Design review of the part built by this model. Coordinates are the model's own, in mm. A direction names the side the tool comes from. Give positions to 0.01 mm unless a question says otherwise; leave off trailing zeros. Order: outer loops, then holes, each group sorted by start corner. A loop starts at its lowest first (then second) coordinate and runs counter-clockwise, first axis right, second up. Notation, with made-up numbers: (86.25, 86.25) - (114.25, 86.25) arc R13 cw to (114.25, 93.25) - close; hole circle Ø7 at (45, 55). An arc over 180 degrees is marked (long way). Write each question's results on one line, items separated by ' | '. Start each with the question number.
Autodesk Inventor part; units mm, degrees
ref_plane "YZ Plane" through (0, 0, 0) normal (1, 0, 0) x (0, 1, 0)
ref_plane "XZ Plane" through (0, 0, 0) normal (0, 1, 0) x (-1, 0, 0)
ref_plane "XY Plane" through (0, 0, 0) normal (0, 0, 1) x (1, 0, 0)
sketch "Skizze1" plane through (0, 0, 0) normal (0, 0, 1) x (1, 0, 0)
  line L0 (-40, -9) -> (40, -9)
  line L1 (40, -9) -> (40, 9)
  line L2 (40, 9) -> (-40, 9)
  line L3 (-40, 9) -> (-40, -9)
  line L4 (-40, -9) -> (40, 9) construction
  line L5 (40, -9) -> (-40, 9) construction
  point P0 (0, 0)
  dimension "Breite" = 80
  dimension "Höhe" = 18
extrude "Extrusion1" add sketch "Skizze1" along normal blind 10
sketch "Skizze2" plane through (0, 0, 10) normal (0, 0, 1) x (1, 0, 0)
  line L0 (40, 9) -> (-40, 9)
  line L1 (-30, -9) -> (30, -9)
  line L2 (30, -9) -> (30, 9)
  line L3 (30, 9) -> (-30, 9)
  line L4 (-30, 9) -> (-30, -9)
  line L5 (-30, -9) -> (30, 9) construction
  line L6 (30, -9) -> (-30, 9) construction
  point P0 (0, 0)
  dimension "Breite_ObererKasten" = 60
extrude "Extrusion2" add sketch "Skizze2" along normal blind 2
sketch "Skizze3" plane through (0, 0, 0) normal (0, 0, -1) x (-1, 0, 0)
  line L0 (0, -12.6) -> (0, 12.6)
  point P0 (0, 0)
  point P1 (-35, 0)
  point P2 (35, 0)
  dimension "Abstand_Bohrung" = 70
hole "Bohrung1" at (35, 0, 0) at (-35, 0, 0) direction (0, 0, 1) diameter 4.5 end through all counterbore diameter 8 counterbore depth 4.6
properties part number "ABI_Kasten"
Q1. Machinability: for faces 1 (the flat face through (37, 2, 4.6)), 2 (the flat face through (-40, 0, 5)), 3 (the flat face through (33.8, 2.1, 10)), 4 (the flat face through (-36.2, 2.1, 10)), which of the approach directions +Z, -Z, +X, -X, +Y, -Y give a long, thin tool a straight path to every point of the face, cutting with its end or side? Answer none if there is none.
Q2. Add section B-B (y = 0). Give the boundary of the cut face in (x, z), plus the area to 3 significant figures.
Q3. Draft analysis for pull direction Y (two halves, no side actions). For faces 5 (the cylindrical face through (32.77, -0.29, 7.34)), 6 (the flat face through (-1, -9, 6)), 7 (the flat face through (0, 0, 12)), state which applies: pulls with the +Y half, pulls with the -Y half, needs draft (parallel to the pull), parting line crosses it, or undercut.
Q4. Add section C-C (z = 7.75). Give the boundary of the cut face in (x, y).
Q5. For line 1 (X direction, y = 0, z = 3.35); line 2 (X direction, y = 0, z = 6.05); line 3 (Y direction, x = 35, z = 7.95), list the stretches that pass through material, from the lowest coordinate up. Write a range as [from, to].
Q6. Insertion check: pin 1 Ø8 at (x, y) = (36, -1.5) entering from +Z; pin 2 Ø4 at (x, y) = (-37, 1) entering from -Z; pin 3 Ø6.5 at (x, y) = (35, 0) entering from -Z; pin 4 Ø1.6 at (y, z) = (1, 11.5) entering from -X. Each pin has a flat end and moves straight along its axis. Give the tip position at first contact, or say it passes through.
Q7. Add section D-D (y = 5.75). Give the boundary of the cut face in (x, z), plus the area to 3 significant figures.
Q8. Add section A-A (x = -35). Give the boundary of the cut face in (y, z).
Verdict:
1) face 1: -Z | face 2: +Z, -Z, -X, +Y, -Y | face 3: +Z, +X, +Y, -Y | face 4: +Z, -X, +Y, -Y
2) outline: (-40, 0) - (-39, 0) - (-39, 4.6) - (-37.25, 4.6) - (-37.25, 10) - (-40, 10) - close; (-32.75, 4.6) - (-31, 4.6) - (-31, 0) - (31, 0) - (31, 4.6) - (32.75, 4.6) - (32.75, 10) - (30, 10) - (30, 12) - (-30, 12) - (-30, 10) - (-32.75, 10) - close; (37.25, 4.6) - (39, 4.6) - (39, 0) - (40, 0) - (40, 10) - (37.25, 10) - close | area: 798 mm2
3) face 5: undercut | face 6: pulls with the -Y half | face 7: needs draft
4) outline: (-40, -9) - (40, -9) - (40, 9) - (-40, 9) - close; hole circle Ø4.5 at (-35, 0); hole circle Ø4.5 at (35, 0)
5) line 1: x = [-40, -39], [-31, 31], [39, 40] | line 2: x = [-40, -37.25], [-32.75, 32.75], [37.25, 40] | line 3: y = [-9, -2.25], [2.25, 9]
6) pin 1: stops at z = 10 | pin 2: stops at z = 0 | pin 3: stops at z = 4.6 | pin 4: stops at x = -30
7) outline: (-40, 0) - (40, 0) - (40, 10) - (30, 10) - (30, 12) - (-30, 12) - (-30, 10) - (-40, 10) - close | area: 920 mm2
8) outline: (-9, 0) - (-4, 0) - (-4, 4.6) - (-2.25, 4.6) - (-2.25, 10) - (-9, 10) - close; (2.25, 4.6) - (4, 4.6) - (4, 0) - (9, 0) - (9, 10) - (2.25, 10) - close
